Could you check a few things on this model? Use its own coordinates, in mm. Coordinates: 2 decimals unless noted, no trailing zeros. Write each loop counter-clockwise with the first axis right and the second up, starting at its lowest first coordinate (ties: lowest second). Pieces come first, ordered by that corner, then holes. Notation, with made-up numbers: M 89,-10.75 L 95,-10.75 A20 cw 95,8.25 Z; hole C 69,67.5 d1. An arc over 180 degrees is marked long. Answer as CSV lines item,"result". Start each with the question number.
Item 1: I'm going to push flat-ended pins straight in: P1, Ø1.6, axis at y = 159, z = 1, coming from the -X side; P2, Ø1, axis at y = 306.5, z = 1.5, coming from the +X side; P3, Ø1.6, axis at x = 311.5, z = 1.5, coming from the +Y side. Where does each tip first touch, or does it pass through?
Item 2: Suppose I cut it at B-B, the plane x = 397. Write out the boundary of the cut face in (y, z) (3 decimals).
Item 3: Suppose I cut it at A-A, the plane y = 208. Write out the boundary of the cut face in (x, z) (3 decimals), and give its area (3 significant figures).
Item 4: We'd pull the mould along X, two halves only. Please class faces 1 (the cylindrical face through (332.269, 285.473, 1.565)), 2 (the flat face through (333, 234, 0)): +X half, -X half, draft (parallel to the pull), parting line (faces both ways), or undercut.
Item 5: Suppose I cut it at C-C, the plane y = 172. Write out the boundary of the cut face in (x, z) (3 decimals), and give its area (3 significant figures).
Item 6: Suppose I cut it at D-D, the plane z = 1.75. State how many separate pieces and enclosed holes the cut face has, and give its area (3 significant figures).
Item 7: If I drill on line 1 along Y through (x, z) = (378, 2.4); line 2 along X through (y, z) = (194, 1.8); line 3 along Y through (x, z) = (404, 2.55), over which ranges is the centre line in solid material (lowest first)? Write a range as [from, to].
```python
from build123d import *

# Parameters (mm, degrees)
SKETCH1_R           = 3.05
SKETCH1_W           = 89.973098965
SKETCH1_H           = 90.646237782
BOSS_EXTRUDE1_DEPTH = 3.175


with BuildPart() as part:
    # Sketch1 → Boss-Extrude1 (new body)
    with BuildSketch(Plane.XY):
        Polygon((311.775650515, 305.698342824), (311.775650515, 289.751882688), (308.79500376, 289.751882688), (308.79500376, 272.936067248), (313.017586662, 272.936067248), (313.017586662, 270.824775797), (313.017586662, 268.713484346), (308.79500376, 268.713484346), (308.79500376, 251.897668907), (311.775650515, 251.897668907), (311.775650515, 214.043455125), (308.79500376, 214.043455125), (308.79500376, 197.227639686), (313.017586662, 197.227639686), (313.017586662, 195.116348235), (313.017586662, 193.005056783), (308.79500376, 193.005056783), (308.79500376, 176.189241344), (311.775650515, 176.189241344), (311.775650515, 160.242781208), (327.722110651, 160.242781208), (327.722110651, 157.262134453), (344.53792609, 157.262134453), (344.53792609, 161.484717355), (346.649217542, 161.484717355), (348.760508993, 161.484717355), (348.760508993, 157.262134453), (365.576324432, 157.262134453), (365.576324432, 160.242781208), (403.430538214, 160.242781208), (403.430538214, 157.262134453), (420.246353653, 157.262134453), (420.246353653, 161.484717355), (422.357645104, 161.484717355), (424.468936555, 161.484717355), (424.468936555, 157.262134453), (441.284751995, 157.262134453), (441.284751995, 160.242781208), (457.231212131, 160.242781208), (457.231212131, 176.189241344), (460.211858886, 176.189241344), (460.211858886, 193.005056783), (455.989275984, 193.005056783), (455.989275984, 195.116348235), (455.989275984, 197.227639686), (460.211858886, 197.227639686), (460.211858886, 214.043455125), (457.231212131, 214.043455125), (457.231212131, 251.897668907), (460.211858886, 251.897668907), (460.211858886, 268.713484346), (455.989275984, 268.713484346), (455.989275984, 270.824775797), (455.989275984, 272.936067248), (460.211858886, 272.936067248), (460.211858886, 289.751882688), (457.231212131, 289.751882688), (457.231212131, 305.698342824), (441.284751995, 305.698342824), (441.284751995, 308.678989579), (424.468936555, 308.678989579), (424.468936555, 304.456406677), (422.357645104, 304.456406677), (420.246353653, 304.456406677), (420.246353653, 308.678989579), (403.430538214, 308.678989579), (403.430538214, 305.698342824), (365.576324432, 305.698342824), (365.576324432, 308.678989579), (348.760508993, 308.678989579), (348.760508993, 304.456406677), (346.649217542, 304.456406677), (344.53792609, 304.456406677), (344.53792609, 308.678989579), (327.722110651, 308.678989579), (327.722110651, 305.698342824), align=None)
        with Locations((334.51688184, 283.411573885)):
            Circle(SKETCH1_R, mode=Mode.SUBTRACT)
        with Locations(Location((434.302437265, 283.655336103, 0), (0, 0, 180))):
            Circle(SKETCH1_R, mode=Mode.SUBTRACT)
        with Locations((434.489980805, 182.765336103)):
            Circle(SKETCH1_R, mode=Mode.SUBTRACT)
        with Locations(Location((334.704655446, 182.517816292, 0), (0, 0, 180))):
            Circle(SKETCH1_R, mode=Mode.SUBTRACT)
        with Locations((384.503431322, 232.970562016)):
            Rectangle(SKETCH1_W, SKETCH1_H, mode=Mode.SUBTRACT)
    extrude(amount=BOSS_EXTRUDE1_DEPTH)


solid = part.part
```
Ans:
1,P1,"stops at x = 327.72"
1,P2,"stops at x = 441.28"
1,P3,"stops at y = 305.7"
2,outline,"M 160.243,0 L 187.647,0 L 187.647,3.175 L 160.243,3.175 Z; M 278.294,0 L 305.698,0 L 305.698,3.175 L 278.294,3.175 Z"
3,outline,"M 308.795,0 L 339.517,0 L 339.517,3.175 L 308.795,3.175 Z; M 429.49,0 L 460.212,0 L 460.212,3.175 L 429.49,3.175 Z"
3,area,"195 mm^2"
4,face 1,"undercut"
4,face 2,"draft"
5,outline,"M 311.776,0 L 457.231,0 L 457.231,3.175 L 311.776,3.175 Z"
5,area,"462 mm^2"
6,separate pieces,"1"
6,enclosed holes,"5"
6,area,"13,600 mm^2"
7,line 1,"y = [160.24, 187.65], [278.29, 305.7]"
7,line 2,"x = [313.02, 339.52], [429.49, 455.99]"
7,line 3,"y = [157.26, 187.65], [278.29, 308.68]"
